```python
from build123d import *

# Parameters (mm, degrees)
IZIM2_R               = 4.25
KES_EKSTR_ZYON1_DEPTH = 30
RADYUS1_R             = 1


with BuildPart() as part:
    # Çizim1 → Döndür1 (revolve)
    with BuildSketch(Plane.XY):
        Polygon((0, 0), (0, 15), (38, 15), (38, 7.5), (46, 7.5), (46, 0), align=None)
    revolve(axis=Axis((46, 0, 0), (-1, 0, 0)))

    # Çizim2 → Kes-Ekstrüzyon1 (cut)
    with BuildSketch(Plane.ZY):
        with Locations(Location((0, 0, 0), (0, 0, 270))):
            Circle(IZIM2_R)
    extrude(amount=-KES_EKSTR_ZYON1_DEPTH, mode=Mode.SUBTRACT)

    # Radyus1
    radyus1_edges = [part.edges().sort_by_distance(p)[0] for p in [
        (46, -7.5, 0),
        (38, -15, 0),
        (0, -15, 0),
    ]]
    fillet(radyus1_edges, radius=RADYUS1_R)


solid = part.part
```
Work out the finished part from the listing and answer in its coordinate system (mm). A direction names the side the tool comes from. Give positions to 0.01 mm unless a question says otherwise; leave off trailing zeros. Loops run counter-clockwise (first coordinate to the right, second up) from the corner with the lowest first, then second, coordinate; pieces in that order, holes last. Notation, with made-up numbers: M 88.5,63.5 L 135.5,63.5 A24 ccw 135.5,85.5 Z; hole C -21.75,84 d9. An arc over 180 degrees is marked long. One line per item, written item: value. Start each with the question number.
1. Determine the mould class of faces 1 (the face through (38, 6, 6)), 2 (the face through (41.549, -7.493, -0.33)), 3 (the face through (30, 0, 0)) for opening direction Y: released by +Y, released by -Y, zero draft, split by the parting line, or undercut.
2. Find section A-A (y = 0). Give the vertices of the cut face in (x, z), and give its area (3 significant figures).
3. Find the intervals of material crossed by probe 1 along Z at (x, y) = (19.75, 0); probe 2 along X at (y, z) = (4, 9.75); probe 3 along X at (y, z) = (2, 2.5), in increasing order.
4. Find section C-C (x = 43.5). Give the vertices of the cut face in (y, z), and give its area (3 significant figures).
5. Find section D-D (x = 6.5). Give the vertices of the cut face in (y, z), and give its area (3 significant figures).
6. Which of the six approach directions +Z, -Z, +X, -X, +Y, -Y give full straight-line access (tool end or side, diameter ignored) to faces 4 (the face through (14.79, 0.553, 4.214)), 5 (the face through (46, 0, 0))?
7. Each of these flat-tipped pins is pushed along its axis until it touches: P1, Ø2.5, axis at y = 2, z = 0.5, coming from the -X side; P2, Ø1, axis at x = 31, y = -2.5, coming from the +Z side; P3, Ø1.5, axis at x = 5.5, y = -1.5, coming from the -Z side; P4, Ø2, axis at x = 40, y = 11.5, coming from the -Z side. Where does it stop, or does it pass through?
Reported:
1. face 1: zero draft
1. face 2: split by the parting line
1. face 3: undercut
2. outline: M 0,-14 A1 ccw 1,-15 L 37,-15 A1 ccw 38,-14 L 38,-7.5 L 45,-7.5 A1 ccw 46,-6.5 L 46,6.5 A1 ccw 45,7.5 L 38,7.5 L 38,14 A1 ccw 37,15 L 1,15 A1 ccw 0,14 L 0,4.25 L 30,4.25 L 30,-4.25 L 0,-4.25 Z
2. area: 1,000 mm²
3. probe 1: z = -15 to -4.25, 4.25 to 15
3. probe 2: x = 0 to 38
3. probe 3: x = 30 to 46
4. outline: C 0,0 d15
4. area: 177 mm²
5. outline: C 0,0 d30; hole C 0,0 d8.5
5. area: 650 mm²
6. face 4: -X
6. face 5: +Z, -Z, +X, +Y, -Y
7. P1: stops at x = 30
7. P2: stops at z = 14.87
7. P3: stops at z = -14.98
7. P4: passes through
